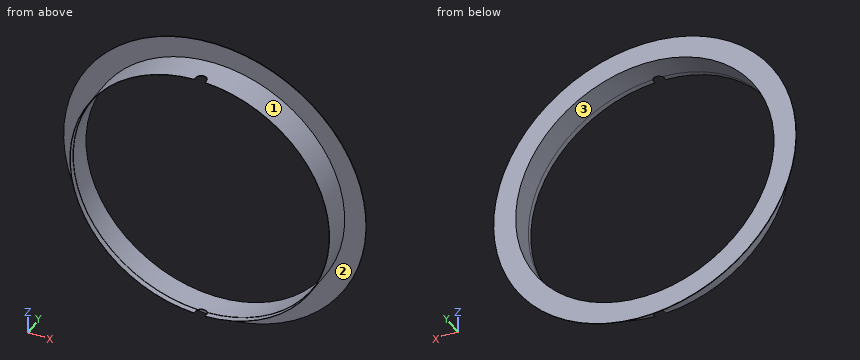
Autodesk Inventor part; units mm, degrees
ref_plane "Work Plane1" through (0, 31.4127, 174.625) normal (0, 0, 1) x (1, 0, 0)
ref_plane "YZ Plane" through (0, 0, 0) normal (1, 0, 0) x (0, 1, 0)
ref_plane "XZ Plane" through (0, 0, 0) normal (0, 1, 0) x (-1, 0, 0)
sketch "Sketch1" plane through (0, 0, 0) normal (1, 0, 0) x (0, 1, 0)
  line L0 (0, 0) -> (0.4853, 0)
  line L1 (3.175, 149.225) -> (31.9024, 149.225)
  line L2 (31.9024, 149.225) -> (31.9024, 174.625)
  line L3 (31.9024, 174.625) -> (31.1086, 174.625)
  line L4 (31.1086, 174.625) -> (31.1087, 150.0187)
  line L5 (31.1087, 150.0187) -> (3.175, 150.0187)
  line L6 (0, 149.225) -> (-3.175, 149.225)
  line L7 (-3.175, 149.6219) -> (3.175, 149.6219)
  line L8 (3.175, 150.0187) -> (-3.175, 150.0187)
  line L9 (-3.175, 150.0187) -> (-3.175, 149.6219)
  line L10 (3.175, 149.6219) -> (3.175, 149.225)
  point P0 (31.4127, 174.625)
  dimension "d0" = 31.9024
  dimension "d1" = 149.225
  dimension "d2" = 25.4
  dimension "d3" = 0.7937
  dimension "d4" = 24.6062
  dimension "d5" = 3.175
  dimension "d6" = 0.3969
revolve "Revolution1" add sketch "Sketch1" angle 360 about axis through (0, 0, 0) along (0, 1, 0)
ref_plane "Work Plane1" through (0, 31.4127, 174.625) normal (0, 0, 1) x (1, 0, 0)
sketch "Sketch2" plane through (0, 31.4127, 174.625) normal (0, 0, 1) x (1, 0, 0)
  line L0 (149.6219, -34.5877) -> (-149.6219, -34.5877)
  arc A0 (6.35, -31.4127) -> (-6.35, -31.4127) centre (0, -31.4127) ccw
  line L1 (-6.35, -34.5877) -> (-6.35, -31.4127)
  line L2 (6.35, -34.5877) -> (6.35, -31.4127)
  line L3 (-6.35, -34.5877) -> (6.35, -34.5877)
  point P0 (0, -31.4127)
  dimension "d10" = 12.7
  dimension "d11" = 0
  dimension "d12" = 3.175
extrude "Extrusion1" cut sketch "Sketch2" against normal through all
properties part number "Layer2_Top"
Build history of the part. All positions in model axes, mm. Face numbers are marked on the shaded views. Coordinates: 2 decimals unless noted, no trailing zeros. Order: outer loops, then holes, each group sorted by start corner. A loop starts at its lowest first (then second) coordinate and runs counter-clockwise, first axis right, second up. Notation, with made-up numbers: (72.25, 82) -> (87.25, 82) arc R19 ccw to (87.25, 98) -> close; hole circle Ø8 at (13.25, 61). An arc over 180 degrees is marked (long way). One line per item, written item: value.
(1) Slice it at C-C, the plane y = 11.5. List the corners of the cut face in (x, z) (3 decimals).
Checked values:
outline: circle Ø300.037 at (0, 0); hole circle Ø298.45 at (0, 0)
(2) Slice it at A-A, the plane x = 0. List the corners of the cut face in (y, z) (3 decimals).
Checked values:
outline: (6.35, -150.019) -> (31.109, -150.019) -> (31.109, -174.625) -> (31.902, -174.625) -> (31.902, -149.225) -> (6.35, -149.225) -> close; (6.35, 149.225) -> (31.902, 149.225) -> (31.902, 174.625) -> (31.109, 174.625) -> (31.109, 150.019) -> (6.35, 150.019) -> close
(3) Drop flat-ended pins along their axis: pin 1 Ø12 at (y, z) = (11, -50.5) entering from -X; pin 2 Ø4 at (x, y) = (67.5, 5.5) entering from -Z; pin 3 Ø6 at (y, z) = (4, -106) entering from +X. Give the stop position or say it passes through.
Checked values:
pin 1: x = -143.27
pin 2: z = -134.96
pin 3: x = 109.07
(4) Probe line 1 (Z direction, x = 0, y = 25) (3 decimals); line 2 (Z direction, x = 57.5, y = 3.5). List the from-to ranges inside material, lowest first. Write a range as [from, to].
Checked values:
line 1: [-150.019, -149.225], [149.225, 150.019]
line 2: [-138.56, -137.7], [137.7, 138.56]
(5) Mould opens along X. For the marked faces 1, 2 and 3 say: pulls with the +X half, pulls with the -X half, needs draft (parallel to the pull), parting line crosses it, or undercut.
Checked values:
face 1: parting line crosses it
face 2: needs draft
face 3: undercut
